Build history of the part. All positions in model axes, mm. Round coordinates to 2 decimals unless told otherwise and drop trailing zeros. Write each loop counter-clockwise with the first axis right and the second up, starting at its lowest first coordinate (ties: lowest second). Pieces come first, ordered by that corner, then holes. Notation, with made-up numbers: M -20,89.25 L 0,89.25 A19 ccw 0,95.25 Z; hole C 77.25,-3 d9. An arc over 180 degrees is marked long. Use a Markdown table: item, result.
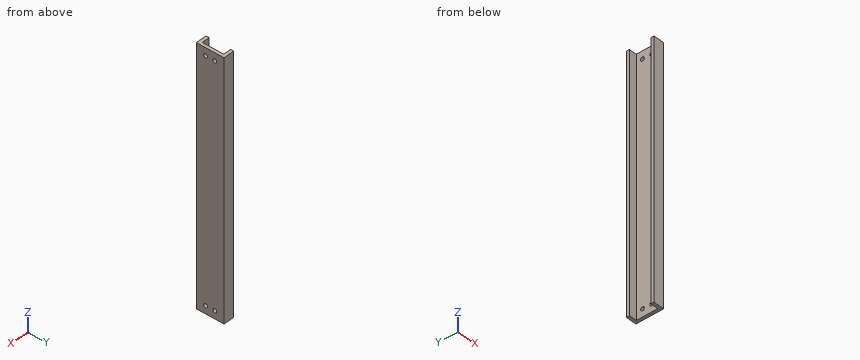
from build123d import *

# Parameters (mm, degrees)
BOSS_EXTRUDE1_DEPTH = 162.5
SKETCH2_R           = 1.25
CUT_EXTRUDE1_DEPTH  = 8


with BuildPart() as part:
    # Sketch1 → Boss-Extrude1 (new body)
    with BuildSketch(Plane.XY):
        Polygon((-7, 9.888282785), (0, 9.888282785), (0, -8.111717215), (-7, -8.111717215), (-7, -6.111717215), (-2, -6.111717215), (-2, 7.888282785), (-7, 7.888282785), align=None)
    extrude(amount=-BOSS_EXTRUDE1_DEPTH)

    # Sketch2 → Cut-Extrude1 (cut, through all)
    with BuildSketch(Plane(origin=(0, 0, 0), x_dir=(0, 0, -1), z_dir=(1, 0, 0))):
        with Locations((5, 3.888282785)):
            Circle(SKETCH2_R)
        with Locations((5, -2.111717215)):
            Circle(SKETCH2_R)
        with Locations((157.5, -2.111717215)):
            Circle(SKETCH2_R)
        with Locations((157.5, 3.888282785)):
            Circle(SKETCH2_R)
    extrude(amount=-CUT_EXTRUDE1_DEPTH, mode=Mode.SUBTRACT)


solid = part.part
Q1. Cut at B-B on z = -37. Give the cut face in (x, y).
Response values:
| item | result |
|---|---|
| outline | M -7,-8.11 L 0,-8.11 L 0,9.89 L -7,9.89 L -7,7.89 L -2,7.89 L -2,-6.11 L -7,-6.11 Z |
Q2. Cut at A-A on x = -4.75. Give the cut face in (y, z), and give its area (3 significant figures).
Response values:
| item | result |
|---|---|
| outline | M -8.11,-162.5 L -6.11,-162.5 L -6.11,0 L -8.11,0 Z; M 7.89,-162.5 L 9.89,-162.5 L 9.89,0 L 7.89,0 Z |
| area | 650 mm2 |
Q3. Drill centre lines: L1, parallel to Y at x = -1.15, z = -157.5; L2, parallel to Y at x = -6, z = -115.5; L3, parallel to X at y = -5.25, z = -33. Where is each one in solid material? Low to high.
Response values:
| item | result |
|---|---|
| L1 | y = -8.11 to -3.36, -0.86 to 2.64, 5.14 to 9.89 |
| L2 | y = -8.11 to -6.11, 7.89 to 9.89 |
| L3 | x = -2 to 0 |
